Verification items for the finished model (mm, model axes). A direction names the side the tool comes from. Coordinates: 2 decimals unless noted, no trailing zeros. Order: outer loops, then holes, each group sorted by start corner. A loop starts at its lowest first (then second) coordinate and runs counter-clockwise, first axis right, second up. Notation, with made-up numbers: (76, 50.5) -> (99, 50.5) arc R24 ccw to (99, 69.5) -> close; hole circle Ø4 at (52.25, 16.25). An arc over 180 degrees is marked (long way). Write item = value, one per line. Start each with the question number.
1. Set-up check for faces 1 (the flat face through (-1, 25.4, 1)), 2 (the flat face through (30, 0, -30)), 3 (the cylindrical face through (-7.945, -241.849, -35.779)): record each of +Z, -Z, +X, -X, +Y, -Y from which the full face is reachable in a straight line by a thin tool's end or side.
2. Thickness scan on line 1 along Z through (x, y) = (0, -310); line 2 along X through (y, z) = (-205, 1.5); line 3 along Y through (x, z) = (10, 53). Record the ranges inside material, lowest first. Write a range as from..to.
3. Go/stop test with flat-tipped pins: P1, Ø6, axis at x = 40, y = -25, coming from the +Z side; P2, Ø1.5, axis at y = -43, z = -38, coming from the -X side; P3, Ø5, axis at x = -41.5, z = 25.5, coming from the -Y side. Record where each tip stops, or that it passes through.
4. Release check for a two-part mould opening along X. For faces 4 (the cylindrical face through (-3.507, -290.5, -15.795)), 5 (the flat face through (27, -101.6, -28)), 6 (the flat face through (0, -177.8, 0)), 7 (the cylindrical face through (-7.97, -47.58, 64.96)) record: +X half, -X half, draft (parallel to the pull), parting line (faces both ways), or undercut.
5. Cross-section at B-B on y = -51. Record the cut outline in (x, z), plus the area to 3 significant figures.
6. Cross-section at A-A on y = -302. Record the cut outline in (x, z), plus the area to 3 significant figures.
from build123d import *

# Parameters (mm, degrees)
F0_R        = 36.650285017
F1_DEPTH    = 50.8
F2_R        = 16.1794098337
F3_DEPTH    = 127
F5_R        = 28.203657399
F5_R_2      = 16.1794098337
F4_R        = 16.1794098337
F3_FACE_R   = 16.1794098337
F6_DEPTH    = 50.8
F7_DEPTH    = 101.6
F8_DEPTH    = 50.8
F9_DEPTH    = 101.6
F10_DEPTH   = 25.4
F11_R       = 67.0391911282
F9_FACE_R   = 36.650285017
F9_FACE_R_2 = 16.1794098337
F12_DEPTH   = 101.6
F13_R       = 20.32
F14_SIZE    = 5.08


with BuildPart() as f1:
    # F0 (on Front) → F1 (new body)
    with BuildSketch(Plane.XZ):
        Circle(F0_R)
    extrude(amount=F1_DEPTH)

    # F2 (on face) → F3 (join)
    with BuildSketch(Plane.XZ.offset(50.8)):
        Circle(F2_R)
    extrude(amount=F3_DEPTH)

    # F5 (on face) + F4 (on face) + F3_face (on face) → F6 (cut)
    with BuildSketch(Plane.XZ.offset(177.8)):
        Circle(F5_R)
        Circle(F5_R_2, mode=Mode.SUBTRACT)
        Circle(F5_R_2)
    with BuildSketch(Plane.XZ.offset(177.8)):
        Circle(F4_R)
    with BuildSketch(Plane.XZ.offset(177.8)):
        Circle(F3_FACE_R)
    extrude(amount=-F6_DEPTH, mode=Mode.SUBTRACT)

    # F7 (add): faces of the model
    f7_faces = [f1.faces().sort_by_distance(p)[0] for p in [
        (-35.6136584143, -50.8, 0),
        (0, 0, 0),
    ]]
    extrude(f7_faces, amount=F7_DEPTH, dir=(0, -1, 0))

    # F8 (add): faces of the model
    f8_faces = [f1.faces().sort_by_distance(p)[0] for p in [
        (-35.6136584143, -152.4, 0),
        (0, -127, 0),
        (0, 0, 0),
    ]]
    extrude(f8_faces, amount=F8_DEPTH, dir=(0, -1, 0))

    # F9 (add): faces of the model
    f9_faces = [f1.faces().sort_by_distance(p)[0] for p in [
        (-35.6136584143, -203.2, 0),
        (0, 0, 0),
    ]]
    extrude(f9_faces, amount=F9_DEPTH, dir=(0, -1, 0))

    # F10 (add): faces of the model
    f10_faces = [f1.faces().sort_by_distance(p)[0] for p in [
        (0, -177.8, 0),
        (0, 0, 0),
    ]]
    extrude(f10_faces, amount=-F10_DEPTH, dir=(0, -1, 0))

    # F11 (on Front) + F9_face (on face) → F12 (join)
    with BuildSketch(Plane.XZ):
        with Locations((0.7551472518, -1.5102935722)):
            Circle(F11_R)
    with BuildSketch(Plane.XZ.offset(304.8)):
        Circle(F9_FACE_R)
        Circle(F9_FACE_R_2, mode=Mode.SUBTRACT)
    extrude(amount=F12_DEPTH)

    # F13
    f13_edges = [f1.edges().sort_by_distance(p)[0] for p in [
        (-36.650285, -406.4, 0),
    ]]
    fillet(f13_edges, radius=F13_R)

    # F14
    f14_edges = [f1.edges().sort_by_distance(p)[0] for p in [
        (-66.284044, -101.6, -1.510294),
    ]]
    chamfer(f14_edges, length=F14_SIZE)


solid = f1.part
Worked out:
q1.face_1 = +Z, -Z, +X, -X, +Y
q1.face_2 = +Y
q1.face_3 = -Y
q2.line_1 = -36.65..-16.18, 16.18..36.65
q2.line_2 = -36.62..-16.11, 16.11..36.62
q2.line_3 = -101.6..0
q3.P1 = 54.89
q3.P2 = -55.96
q3.P3 = -101.6
q4.face_4 = undercut
q4.face_5 = draft
q4.face_6 = undercut
q4.face_7 = parting line
q5.outline = circle Ø134.08 at (0.76, -1.51)
q5.area = 14,100 mm²
q6.outline = circle Ø73.3 at (0, 0); hole circle Ø32.36 at (0, 0)
q6.area = 3,400 mm²
